from build123d import *

# Parameters (mm, degrees)
SKETCH1_W                                       = 320
SKETCH1_H                                       = 320
SKETCH1_R                                       = 2.525
BOSS_EXTRUDE1_DEPTH                             = 6.35
CSK_FOR_M5_FLAT_HEAD_MACHINE_SCREW1_D           = 5.5
CSK_FOR_M5_FLAT_HEAD_MACHINE_SCREW1_DEPTH       = 6.35
CSK_FOR_M5_FLAT_HEAD_MACHINE_SCREW1_CSINK_D     = 10.6
CSK_FOR_M5_FLAT_HEAD_MACHINE_SCREW1_CSINK_ANGLE = 90


with BuildPart() as part:
    # Sketch1 → Boss-Extrude1 (new body)
    with BuildSketch(Plane(origin=(0, 0, 0), x_dir=(1, 0, 0), z_dir=(0, 1, 0))):
        Rectangle(SKETCH1_W, SKETCH1_H)
        with Locations((152, 152)):
            Circle(SKETCH1_R, mode=Mode.SUBTRACT)
        with Locations((-152, -152)):
            Circle(SKETCH1_R, mode=Mode.SUBTRACT)
        with Locations((152, -152)):
            Circle(SKETCH1_R, mode=Mode.SUBTRACT)
        with Locations((-152, 152)):
            Circle(SKETCH1_R, mode=Mode.SUBTRACT)
    extrude(amount=-BOSS_EXTRUDE1_DEPTH)

    # CSK for M5 Flat Head Machine Screw1
    with Locations(Plane(origin=(-152, 0, -152), x_dir=(0, 0, 1), z_dir=(0, 1, 0))):
        with Locations((0, 0), (0, 304), (304, 304), (304, 0)):
            CounterSinkHole(CSK_FOR_M5_FLAT_HEAD_MACHINE_SCREW1_D / 2, CSK_FOR_M5_FLAT_HEAD_MACHINE_SCREW1_CSINK_D / 2, depth=CSK_FOR_M5_FLAT_HEAD_MACHINE_SCREW1_DEPTH, counter_sink_angle=CSK_FOR_M5_FLAT_HEAD_MACHINE_SCREW1_CSINK_ANGLE)


solid = part.part
Input: part model. Units: mm. Frame: model coordinates. Round coordinates to 2 decimals unless told otherwise and drop trailing zeros. Answer as a JSON object with one key per item and string values. Group by question number.
(1) Pin query (flat end, axial travel): P1, Ø4.5, axis at x = 152, z = -152, coming from the -Y side; P2, Ø7, axis at x = -152, z = -152, coming from the +Y side. Return the tip coordinate at first contact, or that it passes through.
(2) Draft query along Z for faces 1 (the face through (152.86, -2.43, -154.74)), 2 (the face through (-2, 0, -2)), 3 (the face through (154.42, -2.43, 150.46)). Return one class per face: released by +Z, released by -Z, zero draft, split by the parting line, or undercut.
(3) Material intervals for probe 1 along X at (y, z) = (-4.2, 152), sorted ascending. Write a range as from..to.
Here are the results:
{
 "1": {"P1": "passes through", "P2": "stops at y = -1.8"},
 "2": {"face 1": "undercut", "face 2": "zero draft", "face 3": "undercut"},
 "3": {"probe 1": "x = -160..-154.75, -149.25..149.25, 154.75..160"}
}
